Geometry: final body of the model. Coordinates: model frame, mm. A direction names the side the tool comes from. Give positions to 0.01 mm unless a question says otherwise; leave off trailing zeros. Loops run counter-clockwise (first coordinate to the right, second up) from the corner with the lowest first, then second, coordinate; pieces in that order, holes last. Notation, with made-up numbers: (23.25, 16) - (30.25, 16) arc R36 cw to (30.25, 52) - close; hole circle Ø10 at (62, -1.5). An arc over 180 degrees is marked (long way). Answer in a Markdown table with one row per item.
from build123d import *

# Parameters (mm, degrees)
SKETCH_1_W          = 10
SKETCH_1_H          = 10
SKETCH_1_W_2        = 8
SKETCH_1_H_2        = 8
EXTRUDE_1_DEPTH     = 294
SKETCH_2_R          = 2.15
CUT_EXTRUDE_1_DEPTH = 295.212508232


with BuildPart() as part:
    # ｽｹｯﾁ1 → 押し出し-薄板1 (new body)
    with BuildSketch(Plane.XY):
        Rectangle(SKETCH_1_W, SKETCH_1_H)
        Rectangle(SKETCH_1_W_2, SKETCH_1_H_2, mode=Mode.SUBTRACT)
    extrude(amount=EXTRUDE_1_DEPTH)

    # ｽｹｯﾁ2 → ｶｯﾄ - 押し出し1 (cut, through all)
    with BuildSketch(Plane(origin=(5, 0, 0), x_dir=(0, 0, -1), z_dir=(1, 0, 0))):
        with Locations(Location((-5, 0, 0), (0, 0, 90))):
            Circle(SKETCH_2_R)
        with Locations(Location((-289, 0, 0), (0, 0, 90))):
            Circle(SKETCH_2_R)
    extrude(amount=-CUT_EXTRUDE_1_DEPTH, mode=Mode.SUBTRACT)


solid = part.part
Q1. Material intervals for line 1 along Z through (x, y) = (4.7, 0); line 2 along Y through (x, z) = (-1.5, 35.5), sorted ascending.
Check values:
| item | result |
|---|---|
| line 1 | 0 to 2.85, 7.15 to 286.85, 291.15 to 294 |
| line 2 | -5 to -4, 4 to 5 |
Q2. Cut plane B-B (x = 2.25). Output: boundary loops of the cut face in (y, z).
Check values:
| item | result |
|---|---|
| outline | (-5, 0) - (-4, 0) - (-4, 294) - (-5, 294) - close; (4, 0) - (5, 0) - (5, 294) - (4, 294) - close |
Q3. Draft query along X for faces 3 (the flat face through (0, -4, 145)), 4 (the flat face through (-5, 0, 145)), 5 (the flat face through (-4.5, 0.1, 0)). Return one class per face: pulls with the +X half, pulls with the -X half, needs draft (parallel to the pull), parting line crosses it, or undercut.
Check values:
| item | result |
|---|---|
| face 3 | undercut |
| face 4 | pulls with the -X half |
| face 5 | needs draft |
Q4. Cut plane A-A (y = 0). Output: boundary loops of the cut face in (x, z).
Check values:
| item | result |
|---|---|
| outline | (-5, 0) - (-4, 0) - (-4, 2.85) - (-5, 2.85) - close; (-5, 7.15) - (-4, 7.15) - (-4, 286.85) - (-5, 286.85) - close; (-5, 291.15) - (-4, 291.15) - (-4, 294) - (-5, 294) - close; (4, 0) - (5, 0) - (5, 2.85) - (4, 2.85) - close; (4, 7.15) - (5, 7.15) - (5, 286.85) - (4, 286.85) - close; (4, 291.15) - (5, 291.15) - (5, 294) - (4, 294) - close |
Q5. Reachability of faces 1 (the flat face through (0, -5, 145)), 2 (the flat face through (4, 0, 145)) from +Z, -Z, +X, -X, +Y, -Y: full face, straight path, thin tool, end or side. Return the list, or none.
Check values:
| item | result |
|---|---|
| face 1 | +Z, -Z, +X, -X, -Y |
| face 2 | +Z, -Z |
Q6. First-contact query: pin 1 (2.5 mm diameter, centred on y = 0, z = 289, fed in from -X); pin 2 (1.5 mm diameter, centred on x = -3.5, y = 2.5, fed in from -Z). Flat tips, straight axial feed; report the tip coordinate or a pass-through.
Check values:
| item | result |
|---|---|
| pin 1 | through |
| pin 2 | z = 0 |
Q7. Cut plane C-C (z = 22). Output: boundary loops of the cut face in (x, y).
Check values:
| item | result |
|---|---|
| outline | (-5, -5) - (5, -5) - (5, 5) - (-5, 5) - close; hole (-4, -4) - (4, -4) - (4, 4) - (-4, 4) - close |
